CAD build for the part. Positions are in the model's coordinates, mm. Face numbers are marked on the shaded views. A direction names the side the tool comes from. Give positions to 0.01 mm unless a question says otherwise; leave off trailing zeros. Loops run counter-clockwise (first coordinate to the right, second up) from the corner with the lowest first, then second, coordinate; pieces in that order, holes last.
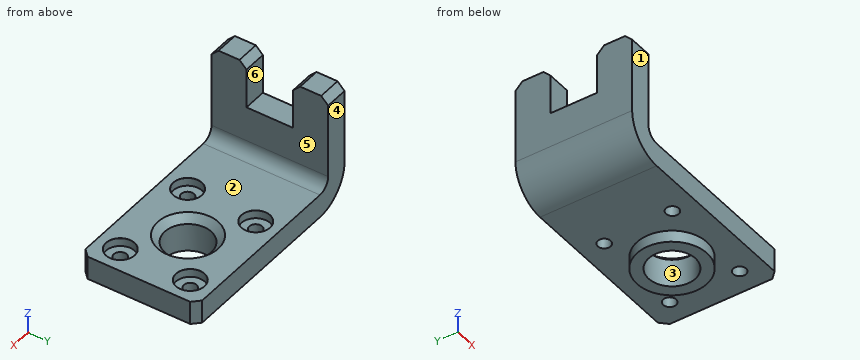
```python
from build123d import *

# Parameters (mm, degrees)
SKETCH1_W                              = 80
SKETCH1_H                              = 50
BOSS_EXTRUDE1_DEPTH                    = 10
SKETCH2_W                              = 50
SKETCH2_H                              = 50
BOSS_EXTRUDE2_DEPTH                    = 10
SKETCH5_W                              = 10
SKETCH5_H                              = 20
CUT_EXTRUDE2_DEPTH                     = 20
SKETCH10_R                             = 15
BOSS_EXTRUDE3_DEPTH                    = 5
SKETCH13_R                             = 10
CUT_EXTRUDE4_DEPTH                     = 15
CHAMFER1_SIZE                          = 3
CBORE_FOR_M5_HEX_HEAD_BOLT2_AT_2_COUNT = 2
CBORE_FOR_M5_HEX_HEAD_BOLT2_AT_2_PITCH = 30
CBORE_FOR_M5_HEX_HEAD_BOLT2_AT_3_COUNT = 2
CBORE_FOR_M5_HEX_HEAD_BOLT2_AT_3_PITCH = 50.908866275
CBORE_FOR_M5_HEX_HEAD_BOLT2_AT_4_COUNT = 2
CBORE_FOR_M5_HEX_HEAD_BOLT2_AT_4_PITCH = 40
CHAMFER2_SIZE                          = 3
CHAMFER3_SIZE                          = 3
CHAMFER4_SIZE                          = 3
FILLET1_R                              = 5
FILLET2_R                              = 15


with BuildPart() as part:
    # Sketch1 → Boss-Extrude1 (new body)
    with BuildSketch(Plane.XY):
        with Locations((40, 25)):
            Rectangle(SKETCH1_W, SKETCH1_H)
    extrude(amount=BOSS_EXTRUDE1_DEPTH)

    # Sketch2 → Boss-Extrude2 (add)
    with BuildSketch(Plane.ZY):
        with Locations((25, 25)):
            Rectangle(SKETCH2_W, SKETCH2_H)
    extrude(amount=BOSS_EXTRUDE2_DEPTH)

    # Sketch5 → Cut-Extrude2 (cut)
    with BuildSketch(Plane.XY.offset(50)):
        with Locations((-5, 25)):
            Rectangle(SKETCH5_W, SKETCH5_H)
    extrude(amount=-CUT_EXTRUDE2_DEPTH, mode=Mode.SUBTRACT)

    # Sketch10 → Boss-Extrude3 (add)
    with BuildSketch(Plane(origin=(0, 0, 0), x_dir=(-1, 0, 0), z_dir=(0, 0, -1))):
        with Locations((-50, 25)):
            Circle(SKETCH10_R)
    extrude(amount=BOSS_EXTRUDE3_DEPTH)

    # Sketch13 → Cut-Extrude4 (cut)
    with BuildSketch(Plane(origin=(0, 0, -5), x_dir=(-1, 0, 0), z_dir=(0, 0, -1))):
        with Locations((-50, 25)):
            Circle(SKETCH13_R)
    extrude(amount=-CUT_EXTRUDE4_DEPTH, mode=Mode.SUBTRACT)

    # Chamfer1
    chamfer1_edges = [part.edges().sort_by_distance(p)[0] for p in [
        (60, 25, 10),
    ]]
    chamfer(chamfer1_edges, length=CHAMFER1_SIZE)

    # Sketch19 → CBORE for M5 Hex Head Bolt2 (revolve, cut)
    with BuildSketch(Plane(origin=(70, 40, 10), x_dir=(0, -1, 0), z_dir=(1, 0, 0))):
        Polygon((0, 0), (0, 15), (2.75, 15), (2.75, 3.5), (6.119, 3.5), (6.119, 0.020977491), (6.144, 0), align=None)
    cbore_for_m5_hex_head_bolt2 = revolve(axis=Axis((70, 40, 16.35), (0, 0, -1)), mode=Mode.SUBTRACT)

    # CBORE for M5 Hex Head Bolt2 at 2: CBORE for M5 Hex Head Bolt2 ×2
    with Locations(*[(0, -i * CBORE_FOR_M5_HEX_HEAD_BOLT2_AT_2_PITCH, 0) for i in range(1, CBORE_FOR_M5_HEX_HEAD_BOLT2_AT_2_COUNT)]):
        add(cbore_for_m5_hex_head_bolt2, mode=Mode.SUBTRACT)

    # CBORE for M5 Hex Head Bolt2 at 3: CBORE for M5 Hex Head Bolt2 ×2
    with Locations(*[Vector(-0.80792282, -0.589288314, 0) * (i * CBORE_FOR_M5_HEX_HEAD_BOLT2_AT_3_PITCH) for i in range(1, CBORE_FOR_M5_HEX_HEAD_BOLT2_AT_3_COUNT)]):
        add(cbore_for_m5_hex_head_bolt2, mode=Mode.SUBTRACT)

    # CBORE for M5 Hex Head Bolt2 at 4: CBORE for M5 Hex Head Bolt2 ×2
    with Locations(*[(-i * CBORE_FOR_M5_HEX_HEAD_BOLT2_AT_4_PITCH, 0, 0) for i in range(1, CBORE_FOR_M5_HEX_HEAD_BOLT2_AT_4_COUNT)]):
        add(cbore_for_m5_hex_head_bolt2, mode=Mode.SUBTRACT)

    # Chamfer2
    chamfer2_edges = [part.edges().sort_by_distance(p)[0] for p in [
        (-5, 50, 50),
    ]]
    chamfer(chamfer2_edges, length=CHAMFER2_SIZE)

    # Chamfer3
    chamfer3_edges = [part.edges().sort_by_distance(p)[0] for p in [
        (-5, 35, 50),
    ]]
    chamfer(chamfer3_edges, length=CHAMFER3_SIZE)

    # Chamfer4
    chamfer4_edges = [part.edges().sort_by_distance(p)[0] for p in [
        (-5, 0, 50),
        (-5, 15, 50),
        (80, 50, 5),
        (80, 0, 5),
    ]]
    chamfer(chamfer4_edges, length=CHAMFER4_SIZE)

    # Fillet1
    fillet1_edges = [part.edges().sort_by_distance(p)[0] for p in [
        (0, 25, 10),
    ]]
    fillet(fillet1_edges, radius=FILLET1_R)

    # Fillet2
    fillet2_edges = [part.edges().sort_by_distance(p)[0] for p in [
        (-10, 25, 0),
    ]]
    fillet(fillet2_edges, radius=FILLET2_R)


solid = part.part
```
1. Probe line 1 along Y through (x, z) = (30, 3.25); line 2 along Z through (x, y) = (19.5, 40); line 3 along X through (y, z) = (40, 8.5). List the from-to ranges inside material, lowest first.
Responses:
line 1: y = 0 to 7.49, 12.51 to 37.25, 42.75 to 50
line 2: z = 0 to 10
line 3: x = -8.52 to 23.88, 36.12 to 63.88, 76.12 to 80
2. Drop flat-ended pins along their axis: pin 1 (10 mm diameter, centred on y = 41, z = 6.5, fed in from -X); pin 2 (14 mm diameter, centred on x = 30, y = 40, fed in from -Z); pin 3 (6 mm diameter, centred on x = 20.5, z = 12.5, fed in from +Y); pin 4 (25 mm diameter, centred on x = 48.5, y = 28.5, fed in from +Z). Give the stop position or say it passes through.
Responses:
pin 1: stops at x = -9.59
pin 2: stops at z = 0
pin 3: stops at y = 50
pin 4: stops at z = 10
3. Saw through at A-A, the plane x = 50. List the corners of the cut face in (y, z), and give its area (3 significant figures).
Responses:
outline: (0, 0) - (10, 0) - (10, -5) - (15, -5) - (15, 7) - (12, 10) - (0, 10) - close; (35, -5) - (40, -5) - (40, 0) - (50, 0) - (50, 10) - (38, 10) - (35, 7) - close
area: 341 mm2
4. Saw through at D-D, the plane x = -3.5. List the corners of the cut face in (y, z).
Responses:
outline: (0, 2.64) - (50, 2.64) - (50, 47) - (47, 50) - (38, 50) - (35, 47) - (35, 30) - (15, 30) - (15, 47) - (12, 50) - (3, 50) - (0, 47) - close
5. Saw through at C-C, the plane x = 70. Count the separate pieces of the cut face and the enclosed holes in it, and give its area (3 significant figures).
Responses:
separate pieces: 3
enclosed holes: 0
area: 343 mm2
6. Saw through at B-B, the plane y = 25. List the corners of the cut face in (x, z), and give its area (3 significant figures).
Responses:
outline: (-10, 15) arc R15 ccw to (5, 0) - (35, 0) - (35, -5) - (40, -5) - (40, 7) - (37, 10) - (5, 10) arc R5 cw to (0, 15) - (0, 30) - (-10, 30) - close; (60, -5) - (65, -5) - (65, 0) - (80, 0) - (80, 10) - (63, 10) - (60, 7) - close
area: 898 mm2
7. Pull direction Y, two halves, no side cores. Call the marked faces 1, 2 and 3: released by +Y, released by -Y, zero draft, split by the parting line, or undercut.
Responses:
face 1: released by -Y
face 2: zero draft
face 3: undercut
8. Tool access for the marked faces 4, 5 and 6: list every direction of +Z, -Z, +X, -X, +Y, -Y with a clear straight run to the whole face (end or side of a thin tool).
Responses:
face 4: +Z, -Z, +X, -X, +Y
face 5: +Z, +X, +Y, -Y
face 6: +Z, +X, -X
